Part model, mm, in its own coordinate system. Face numbers are marked on the shaded views. A direction names the side the tool comes from. Coordinates: 2 decimals unless noted, no trailing zeros. Write each loop counter-clockwise with the first axis right and the second up, starting at its lowest first coordinate (ties: lowest second). Pieces come first, ordered by that corner, then holes. Notation, with made-up numbers: (40.25, 5.5) -> (61.25, 5.5) arc R11 cw to (61.25, 14.5) -> close; hole circle Ø7 at (72.25, -4). An arc over 180 degrees is marked (long way). Write item = value, one per line.
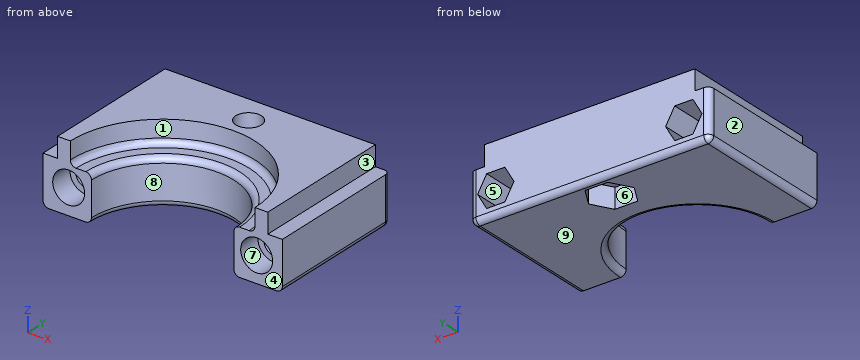
from build123d import *

# Parameters (mm, degrees)
F0_W      = 42
F0_H      = 24.9
F1_DEPTH  = 12
F3_DEPTH  = 4
F5_DEPTH  = 8
F7_D      = 4.5
F8_W      = 2.55
F8_H      = 3.5
F9_DEPTH  = 24.9
F12_D     = 3.5
F14_DEPTH = 3.5
F15_R     = 2.8
F15_R_2   = 1.75
F16_DEPTH = 4
F17_R     = 1.75
F18_DEPTH = 12
F19_R     = 1


# Not quite as in the source:
# - a pattern or mirror of a feature is missing from the dataset's text; its kind, count and spacing are read off the source's solid


with BuildPart() as f1:
    # F0 (on Top) → F1 (new body)
    with BuildSketch(Plane.XY):
        with Locations((0, 12.45)):
            Rectangle(F0_W, F0_H)
    extrude(amount=F1_DEPTH)

    # F2 (on face) → F3 (cut)
    with BuildSketch(Plane.XY.offset(12)):
        with BuildLine():
            Line((-16.2, 0), (16.2, 0))
            ThreePointArc((16.2, 0), (0, 16.2), (-16.2, 0))
        make_face()
    extrude(amount=-F3_DEPTH, mode=Mode.SUBTRACT)

    # F4 (on face) → F5 (cut, through all)
    with BuildSketch(Plane.XY.offset(8)):
        with BuildLine():
            Line((-12.5, 0), (12.5, 0))
            ThreePointArc((12.5, 0), (0, 12.5), (-12.5, 0))
        make_face()
    extrude(amount=-F5_DEPTH, mode=Mode.SUBTRACT)

    # F7 (through all)
    with Locations(Plane.XY.offset(12)):
        with Locations((0, 19.9)):
            Hole(F7_D / 2)

    # F8 (on face) → F9 (cut, through all)
    with BuildSketch(Plane.XZ):
        with Locations((-19.725, 10.25)):
            Rectangle(F8_W, F8_H)
    f9 = extrude(amount=-F9_DEPTH, mode=Mode.SUBTRACT)

    # F9_copies: F9 across plane
    add(f9.mirror(Plane(origin=(0, 0, 0), x_dir=(0, 0, 1), z_dir=(1, 0, 0))), mode=Mode.SUBTRACT)

    # F12 (through all)
    with Locations(Plane.XZ):
        with Locations((-16.5, 4.5), (16.5, 4.5)):
            Hole(F12_D / 2)

    # F13 (on face) → F14 (cut)
    with BuildSketch(Plane.XY):
        Polygon((-2.0005186827, 23.365), (-4.0010373655, 19.9), (-2.0005186827, 16.435), (2.0005186827, 16.435), (4.0010373655, 19.9), (2.0005186827, 23.365), align=None)
    extrude(amount=F14_DEPTH, mode=Mode.SUBTRACT)

    # F15 (on face) → F16 (cut)
    with BuildSketch(Plane.XZ):
        with Locations((16.5, 4.5)):
            Circle(F15_R)
        with Locations((16.5, 4.5)):
            Circle(F15_R_2, mode=Mode.SUBTRACT)
    f16 = extrude(amount=-F16_DEPTH, mode=Mode.SUBTRACT)

    # F16_copies: F16 across plane
    add(f16.mirror(Plane(origin=(0, 0, 0), x_dir=(0, 0, -1), z_dir=(-1, 0, 0))), mode=Mode.SUBTRACT)

    # F17 (on face) → F18 (cut)
    with BuildSketch(Plane(origin=(0, 24.9, 0), x_dir=(-1, 0, 0), z_dir=(0, 1, 0))):
        Polygon((-19.6927469886, 4.5), (-18.0963734943, 1.735), (-14.9036265057, 1.735), (-13.3072530114, 4.5), (-14.9036265057, 7.265), (-18.0963734943, 7.265), align=None)
        with Locations((-16.5, 4.5)):
            Circle(F17_R, mode=Mode.SUBTRACT)
    f18 = extrude(amount=-F18_DEPTH, mode=Mode.SUBTRACT)

    # F18_copies: F18 across plane
    add(f18.mirror(Plane(origin=(0, 0, 0), x_dir=(0, 0, -1), z_dir=(-1, 0, 0))), mode=Mode.SUBTRACT)

    # F19
    f19_edges = [f1.edges().sort_by_distance(p)[0] for p in [
        (21, 24.9, 4.25),
        (0, 24.9, 0),
        (-21, 24.9, 4.25),
        (-21, 12.45, 0),
        (21, 12.45, 0),
        (0, 12.5, 0),
        (0, 12.5, 8),
        (0, 16.2, 8),
    ]]
    fillet(f19_edges, radius=F19_R)


solid = f1.part
Q1. Pin check, flat tips, straight feed: pin 1 (0.8 mm diameter, centred on x = 20.5, y = 7, fed in from +Z); pin 2 (3 mm diameter, centred on x = 17.5, z = 5, fed in from +Y); pin 3 (3 mm diameter, centred on x = -16.5, z = 4.5, fed in from -Y); pin 4 (1.8 mm diameter, centred on y = 6.5, z = 10.5, fed in from +X). Stop position of each tip, or through.
Model answer:
pin_1 = 8.5
pin_2 = 12.9
pin_3 = through
pin_4 = 18.45
Q2. Mould opens along X. For the marked faces 1, 2, 3 and 4 say: released by +X, released by -X, zero draft, split by the parting line, or undercut.
Model answer:
face_1 = undercut
face_2 = released by -X
face_3 = released by +X
face_4 = zero draft
Q3. Probe line 1 (X direction, y = 9, z = 4.75); line 2 (Y direction, x = 0, z = 9.25); line 3 (X direction, y = 7, z = 4.5). List the from-to ranges inside material, lowest first. Write a range as from..to.
Model answer:
line_1 = -21..-18.23, -14.77..-8.67, 8.67..14.77, 18.23..21
line_2 = 16.2..17.65, 22.15..24.9
line_3 = -21..-18.25, -14.75..-10.36, 10.36..14.75, 18.25..21
Q4. Saw through at A-A on x = 0. Give the cut face in (y, z) (3 decimals), and give its area (3 significant figures).
Model answer:
outline = (12.5, 1) arc R1 ccw to (13.5, 0) -> (16.435, 0) -> (16.435, 3.5) -> (17.65, 3.5) -> (17.65, 12) -> (16.2, 12) -> (16.2, 9) arc R1 cw to (15.2, 8) -> (13.5, 8) arc R1 ccw to (12.5, 7) -> close; (22.15, 3.5) -> (23.365, 3.5) -> (23.365, 0) -> (23.9, 0) arc R1 ccw to (24.9, 1) -> (24.9, 12) -> (22.15, 12) -> close
area = 71.1 mm²
Q5. Which spindle directions (+Z, -Z, +X, -X, +Y, -Y) get a long thin tool onto all of the face, cutting with end or side? Do the marked faces 5, 6, 7, 8 and 9. Say none if no direction does.
Model answer:
face_5 = +Y
face_6 = -Z
face_7 = -Y
face_8 = +Z, -Z, -Y
face_9 = -Z, +X, -X, +Y, -Y
Q6. Saw through at B-B on y = 21. Count the separate pieces of the cut face and the enclosed holes in it, and give its area (3 significant figures).
Model answer:
separate_pieces = 2
enclosed_holes = 2
area = 376 mm²
Q7. Saw through at D-D on z = 10.75. Give the cut face in (x, y), and give its area (3 significant figures).
Model answer:
outline = (-18.45, 0) -> (-16.2, 0) arc R16.2 cw to (16.2, 0) -> (18.45, 0) -> (18.45, 24.9) -> (-18.45, 24.9) -> close; hole circle Ø4.5 at (0, 19.9)
area = 491 mm²
